```python
from build123d import *

# Parameters (mm, degrees)
F1_DEPTH = 2.0066
F3_DEPTH = 2
F5_DEPTH = 25.4


with BuildPart() as f1:
    # F0 (on Top) → F1 (new body)
    with BuildSketch(Plane.XY):
        Polygon((-24.6424870433, 43.8434540713), (-50.2907885371, 0.5807072437), (-25.6483014937, -43.2627468276), (24.6424870433, -43.8434540713), (50.2907885371, -0.5807072437), (25.6483014937, 43.2627468276), align=None)
    extrude(amount=F1_DEPTH)

    # F2 (on face) → F3 (join)
    with BuildSketch(Plane.XY.offset(2.0066)):
        Polygon((14.4355614638, 25.0031258911), (-14.4355614638, 25.0031258911), (-28.8711229276, 0), (-14.4355614638, -25.0031258911), (14.4355614638, -25.0031258911), (28.8711229276, 0), align=None)
    extrude(amount=F3_DEPTH)

    # F4 (on face) → F5 (join)
    with BuildSketch(Plane.XY.offset(2.0066)):
        Polygon((8.3927677802, 14.5367002115), (-8.3927677802, 14.5367002115), (-16.7855355604, 0), (-8.3927677802, -14.5367002115), (8.3927677802, -14.5367002115), (16.7855355604, 0), align=None)
        with BuildLine():
            Line((12.8234216162, 43.4108355902), (-11.8176071658, 43.6953653087))
            ThreePointArc((-11.8176071658, 43.6953653087), (0.3606423659, 31.2325860584), (12.8234216162, 43.4108355902))
        make_face()
        with BuildLine():
            ThreePointArc((12.8234216162, 43.4108355902), (12.8240376181, 43.4819668344), (12.8242429543, 43.5531004494))
            ThreePointArc((12.8242429543, 43.5531004494), (0.5740408403, 55.8742308423), (-11.8176071658, 43.6953653087))
            Line((-11.8176071658, 43.6953653087), (12.8234216162, 43.4108355902))
        make_face()
    extrude(amount=F5_DEPTH)


solid = f1.part
```
Read the model definition and answer for the solid it produces. Units are mm, in the model's axes. A direction names the side the tool comes from. Give positions to 0.01 mm unless a question says otherwise; leave off trailing zeros. Loops run counter-clockwise (first coordinate to the right, second up) from the corner with the lowest first, then second, coordinate; pieces in that order, holes last.
Item 1: The part is cut by section D-D (y = -20). Write down the section's boundary in (x, z), and give its area (3 significant figures).
Item 2: The mould has two halves that part along Y. Classify faces 6 (the flat face through (-21.754, -12.327, 2.993)), 7 (the flat face through (-12.53, 7.37, 15.54)), 8 (the flat face through (-1, 1, 0)): released by +Y, released by -Y, zero draft, split by the parting line, or undercut.
Item 3: The part is cut by section B-B (y = 3). Write down the section's boundary in (x, z).
Item 4: The part is cut by section A-A (z = 10.5). Write down the section's boundary in (x, y).
Item 5: Each of these flat-tipped pins is pushed along its axis until it touches: pin 1 Ø3.5 at (x, y) = (2.5, 47) entering from -Z; pin 2 Ø10 at (x, y) = (22.5, 12) entering from +Z; pin 3 Ø1.6 at (x, z) = (-3.5, 2.5) entering from +Y. Where does it stop, or does it pass through?
Item 6: The part is cut by section C-C (x = 23). Write down the section's boundary in (y, z), and give its area (3 significant figures).
Item 7: For faces 1 (the flat face through (-12.648, -7.167, 15.543)), 2 (the flat face through (21.55, -12.68, 2.99)), 3 (the flat face through (21.754, 12.327, 2.993)), 4 (the flat face through (12.648, 7.167, 15.543)), 5 (the flat face through (-21.55, 12.68, 2.99)), determine the directions among +Z, -Z, +X, -X, +Y, -Y from which every point of the face is accessible in a straight line to the end or side of a thin tool.
Item 8: Find the intervals of material crossed by line 1 along Z through (x, y) = (-38.5, -12.5); line 2 along Z through (x, y) = (-15, -18); line 3 along X through (y, z) = (43, 14.75), in increasing order.
Taken from the geometry:
1. outline: (-38.72, 0) - (38.78, 0) - (38.78, 2.01) - (17.32, 2.01) - (17.32, 4.01) - (-17.32, 4.01) - (-17.32, 2.01) - (-38.72, 2.01) - close
1. area: 225 mm2
2. face 6: released by -Y
2. face 7: undercut
2. face 8: zero draft
3. outline: (-48.86, 0) - (48.28, 0) - (48.28, 2.01) - (27.14, 2.01) - (27.14, 4.01) - (15.05, 4.01) - (15.05, 27.41) - (-15.05, 27.41) - (-15.05, 4.01) - (-27.14, 4.01) - (-27.14, 2.01) - (-48.86, 2.01) - close
4. outline: (-16.79, 0) - (-8.39, -14.54) - (8.39, -14.54) - (16.79, 0) - (8.39, 14.54) - (-8.39, 14.54) - close; (12.82, 43.41) arc R12.32 ccw to (12.82, 43.55) arc R12.32 ccw (long way) to start
5. pin 1: stops at z = 2.01
5. pin 2: stops at z = 4.01
5. pin 3: stops at y = 55.45
6. outline: (-43.82, 0) - (43.29, 0) - (43.29, 2.01) - (10.17, 2.01) - (10.17, 4.01) - (-10.17, 4.01) - (-10.17, 2.01) - (-43.82, 2.01) - close
6. area: 215 mm2
7. face 1: +Z, -X, -Y
7. face 2: +Z, +X, -Y
7. face 3: +Z, +X, +Y
7. face 4: +Z, +X
7. face 5: +Z, -X, +Y
8. line 1: z = 0 to 2.01
8. line 2: z = 0 to 4.01
8. line 3: x = -11.81 to 12.81
